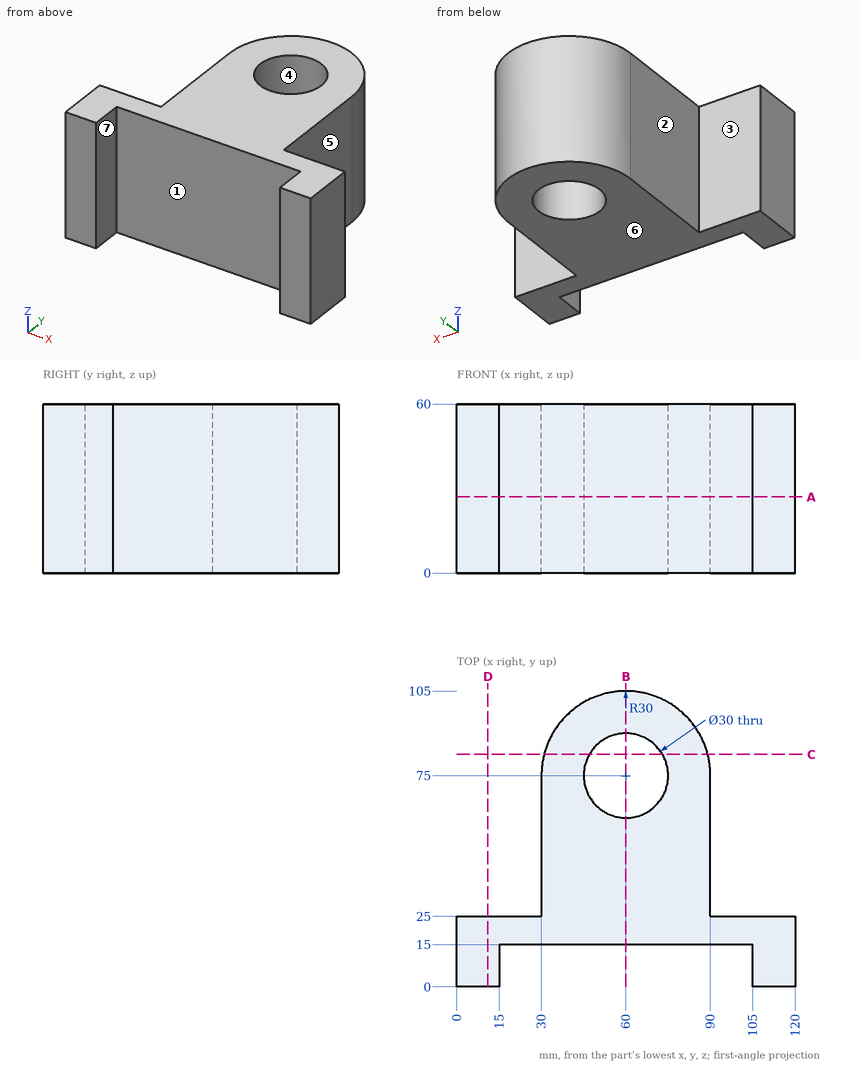
Verification items for this drawing (mm, ordinates from the low corner). A direction names the side the tool comes from. Give positions to 0.01 mm unless a question says otherwise; leave off trailing zeros. Write each loop counter-clockwise with the first axis right and the second up, starting at its lowest first coordinate (ties: lowest second). Pieces come first, ordered by that corner, then holes.
1) Release check for a two-part mould opening along Y. For the marked faces 1, 2, 3 and 4 record: released by +Y, released by -Y, zero draft, split by the parting line, or undercut.
Values follow:
face 1: released by -Y
face 2: zero draft
face 3: released by +Y
face 4: undercut
2) Cross-section at D-D (x = 11). Record the boundary of the cut face in (y, z).
Values follow:
outline: (0, 0) - (25, 0) - (25, 60) - (0, 60) - close
3) Cross-section at B-B (x = 60). Record the boundary of the cut face in (y, z), plus the area to 3 significant figures.
Values follow:
outline: (15, 0) - (60, 0) - (60, 60) - (15, 60) - close; (90, 0) - (105, 0) - (105, 60) - (90, 60) - close
area: 3,600 mm2
4) Set-up check for the marked faces 5, 6 and 7: record each of +Z, -Z, +X, -X, +Y, -Y from which the full face is reachable in a straight line by a thin tool's end or side.
Values follow:
face 5: +Z, -Z, +X, +Y
face 6: -Z, +X, -X, +Y, -Y
face 7: +Z, -Z, -Y
5) Thickness scan on line 1 (Y direction, x = 60, z = 36); line 2 (X direction, y = 9, z = 40); line 3 (X direction, y = 34.5, z = 3). Record the ranges inside material, lowest first.
Values follow:
line 1: y = 15 to 60, 90 to 105
line 2: x = 0 to 15, 105 to 120
line 3: x = 30 to 90
6) Cross-section at A-A (z = 27). Record the boundary of the cut face in (x, y).
Values follow:
outline: (0, 0) - (15, 0) - (15, 15) - (105, 15) - (105, 0) - (120, 0) - (120, 25) - (90, 25) - (90, 75) arc R30 ccw to (30, 75) - (30, 25) - (0, 25) - close; hole circle Ø30 at (60, 75)
7) Go/stop test with flat-tipped pins: pin 1 Ø4 at (y, z) = (80.5, 7) entering from -X; pin 2 Ø25 at (y, z) = (39, 31.5) entering from +X; pin 3 Ø1.5 at (x, z) = (94, 50.5) entering from -Y. Record where each tip stops, or that it passes through.
Values follow:
pin 1: stops at x = 30.2
pin 2: stops at x = 90
pin 3: stops at y = 15
8) Cross-section at C-C (y = 82.5). Record the boundary of the cut face in (x, z), plus the area to 3 significant figures.
Values follow:
outline: (30.95, 0) - (47.01, 0) - (47.01, 60) - (30.95, 60) - close; (72.99, 0) - (89.05, 0) - (89.05, 60) - (72.99, 60) - close
area: 1,930 mm2
